Read the model definition and answer for the solid it produces. Units are mm, in the model's axes. Face numbers are marked on the shaded views. A direction names the side the tool comes from. Coordinates: 2 decimals unless noted, no trailing zeros. Order: outer loops, then holes, each group sorted by start corner. A loop starts at its lowest first (then second) coordinate and runs counter-clockwise, first axis right, second up.
Autodesk Fusion 360 part; units mm, degrees
sketch "Sketch1" plane through (0, 0, 0) normal (0, 0, 1) x (1, 0, 0)
  circle A0 centre (0, 0) radius 20
  circle A1 centre (0, 0) radius 18.4
  circle A2 centre (0, 0) radius 12.4
  circle A3 centre (0, 0) radius 16.8
  dimension "d1" = 40
  dimension "d2" = -1.6
  dimension "d3" = -7.6
  dimension "d4" = -3.2
extrude "Extrude1" add sketch "Sketch1" against normal blind 6.4 contours A0 | A1
extrude "Extrude2" add sketch "Sketch1" against normal blind 1.2 contours A3
extrude "Extrude3" add sketch "Sketch1" along normal blind 9.2 contours A0
extrude "Extrude4" add 1 faces at (19.3922, -0.9936, 9.2) along direction (0, 0, 1) blind 5
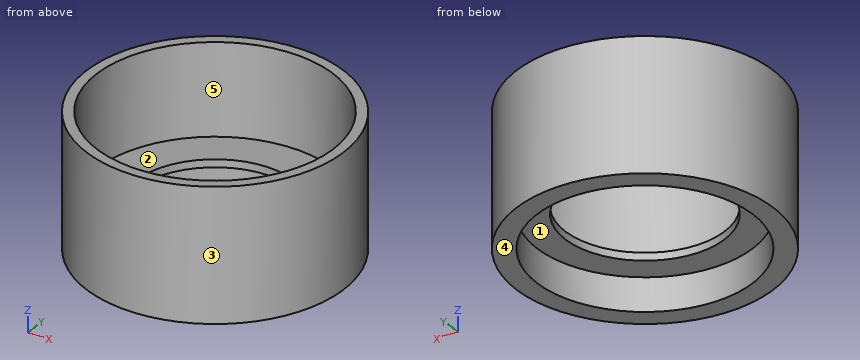
1) A cutting plane is placed at C-C, the plane z = 6.25. Determine the outline of the cut face in (x, y), and give its area (3 significant figures).
A:
outline: circle Ø40 at (0, 0); hole circle Ø36.8 at (0, 0)
area: 193 mm2
2) A cutting plane is placed at A-A, the plane x = 0. Determine the outline of the cut face in (y, z), and give its area (3 significant figures).
A:
outline: (-20, -6.4) - (-16.8, -6.4) - (-16.8, -1.2) - (-12.4, -1.2) - (-12.4, 0) - (-18.4, 0) - (-18.4, 14.2) - (-20, 14.2) - close; (12.4, -1.2) - (16.8, -1.2) - (16.8, -6.4) - (20, -6.4) - (20, 14.2) - (18.4, 14.2) - (18.4, 0) - (12.4, 0) - close
area: 97.0 mm2
3) Determine the mould class of the marked faces 3, 4 and 5 for opening direction Y: pulls with the +Y half, pulls with the -Y half, needs draft (parallel to the pull), parting line crosses it, or undercut.
A:
face 3: parting line crosses it
face 4: needs draft
face 5: undercut
4) A cutting plane is placed at D-D, the plane y = 13. Determine the outline of the cut face in (x, z).
A:
outline: (-15.2, -6.4) - (-10.64, -6.4) - (-10.64, -1.2) - (10.64, -1.2) - (10.64, -6.4) - (15.2, -6.4) - (15.2, 14.2) - (13.02, 14.2) - (13.02, 0) - (-13.02, 0) - (-13.02, 14.2) - (-15.2, 14.2) - close
5) Flat-ended cylindrical pins translate along their axes: pin 1 Ø5 at (x, z) = (-11.5, 1.5) entering from -Y; pin 2 Ø1.5 at (y, z) = (-5, -1) entering from +X; pin 3 Ø1 at (x, y) = (-12, -9.5) entering from +Z. Find the tip coordinate at first contact, or state that the pin passes through.
A:
pin 1: stops at y = -17.86
pin 2: stops at x = 19.54
pin 3: stops at z = 0
6) Which of the six approach directions +Z, -Z, +X, -X, +Y, -Y give full straight-line access (tool end or side, diameter ignored) to the marked faces 1 and 2?
A:
face 1: -Z
face 2: +Z
7) Straight lines are drawn through the part: line 1 (Y direction, x = 0, z = 11); line 2 (Y direction, x = 0, z = -2.8); line 3 (Z direction, x = -6, y = 13.5). For each, find the intervals that lie inside material, in ascending order.
A:
line 1: y = -20 to -18.4, 18.4 to 20
line 2: y = -20 to -16.8, 16.8 to 20
line 3: z = -1.2 to 0
